Build history of the part. All positions in model axes, mm. Face numbers are marked on the shaded views. A direction names the side the tool comes from. Round coordinates to 2 decimals unless told otherwise and drop trailing zeros. Write each loop counter-clockwise with the first axis right and the second up, starting at its lowest first coordinate (ties: lowest second). Pieces come first, ordered by that corner, then holes. Notation, with made-up numbers: (14, 12) - (38, 12) arc R16 ccw to (38, 25) - close; hole circle Ø4 at (16.25, 69). An arc over 180 degrees is marked (long way). Write each question's results on one line, items separated by ' | '.
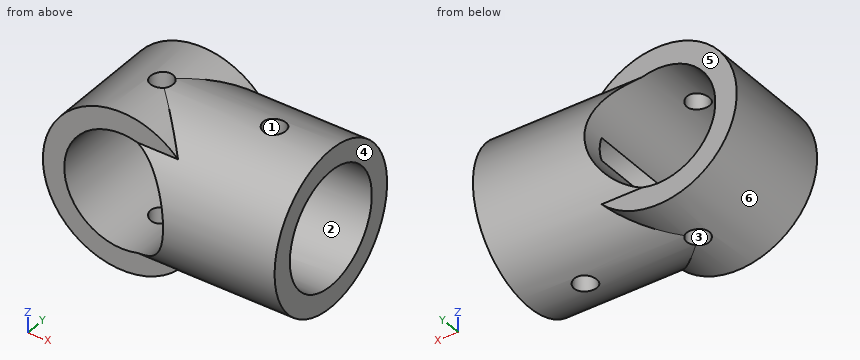
from build123d import *

# Parameters (mm, degrees)
CYLINDER001_R          = 10.2
CYLINDER001_DEPTH      = 20
CYLINDER002_R          = 2
CYLINDER002_DEPTH      = 30
CYLINDER003_R          = 2
CYLINDER003_DEPTH      = 30
CYLINDER_R             = 10.2
CYLINDER_DEPTH         = 30
CYLINDER_ROLL_ANGLE    = -90
CYLINDER004_R          = 14
CYLINDER004_DEPTH      = 30
CYLINDER005_R          = 14
CYLINDER005_DEPTH      = 20
CYLINDER005_ROLL_ANGLE = -90


with BuildPart() as cylinder001:
    # Cylinder001 → Cylinder001 (new body)
    with BuildSketch(Plane(origin=(10, 0, 0), x_dir=(0, -1, 0), z_dir=(1, 0, 0))):
        Circle(CYLINDER001_R)
    extrude(amount=CYLINDER001_DEPTH)


with BuildPart() as cylinder002:
    # Cylinder002 → Cylinder002 (new body)
    with BuildSketch(Plane.XY.offset(-15)):
        Circle(CYLINDER002_R)
    extrude(amount=CYLINDER002_DEPTH)


with BuildPart() as cylinder003:
    # Cylinder003 → Cylinder003 (new body)
    with BuildSketch(Plane(origin=(20, 0, -15), x_dir=(1, 0, 0), z_dir=(0, 0, 1))):
        Circle(CYLINDER003_R)
    extrude(amount=CYLINDER003_DEPTH)


with BuildPart() as negative_fusion:
    # Cylinder → Cylinder (new body)
    with BuildSketch(Plane.XY):
        Circle(CYLINDER_R)
    extrude(amount=CYLINDER_DEPTH)


with BuildPart() as negative_fusion_1:
    # Cylinder roll: moved
    add(negative_fusion.part.rotate(Axis((0, 0, 0), (1, 0, 0)), CYLINDER_ROLL_ANGLE))


with BuildPart() as negative_fusion_2:
    # Cylinder placement: moved
    add(negative_fusion_1.part.moved(Location((0, -15, 0))))

    # Fusion: union Cylinder001, Cylinder002, Cylinder003
    add(cylinder001.part)
    add(cylinder002.part)
    add(cylinder003.part)


with BuildPart() as cylinder004:
    # Cylinder004 → Cylinder004 (new body)
    with BuildSketch(Plane(origin=(0, 0, 0), x_dir=(0, -1, 0), z_dir=(1, 0, 0))):
        Circle(CYLINDER004_R)
    extrude(amount=CYLINDER004_DEPTH)


with BuildPart() as cut:
    # Cylinder005 → Cylinder005 (new body)
    with BuildSketch(Plane.XY):
        Circle(CYLINDER005_R)
    extrude(amount=CYLINDER005_DEPTH)


with BuildPart() as cut_1:
    # Cylinder005 roll: moved
    add(cut.part.rotate(Axis((0, 0, 0), (1, 0, 0)), CYLINDER005_ROLL_ANGLE))


with BuildPart() as cut_2:
    # Cylinder005 placement: moved
    add(cut_1.part.moved(Location((0, -10, 0))))

    # Fusion001: union Cylinder004
    add(cylinder004.part)

    # Cut: cut Negative Fusion
    add(negative_fusion_2.part, mode=Mode.SUBTRACT)


solid = cut_2.part
(1) Slice it at D-D, the plane z = -11. Write the cut outline in (x, y), and give its area (3 significant figures).
Worked answers:
outline: (-8.66, -10) - (8.66, -10) - (8.66, -8.66) - (30, -8.66) - (30, 8.66) - (8.66, 8.66) - (8.66, 10) - (-8.66, 10) - close; hole circle Ø4 at (0, 0); hole circle Ø4 at (20, 0) | area: 691 mm2
(2) Slice it at C-C, the plane y = 0. Write the cut outline in (x, z), and give its area (3 significant figures).
Worked answers:
outline: (-2, -13.86) - (-2, -10) arc R10.2 cw to (-2, 10) - (-2, 13.86) arc R14 ccw to start; (2, -14) - (18, -14) - (18, -10.2) - (10, -10.2) - (10, -2.01) arc R10.2 cw to (2, -10) - close; (2, 10) arc R10.2 cw to (10, 2.01) - (10, 10.2) - (18, 10.2) - (18, 14) - (2, 14) - close; (22, -14) - (30, -14) - (30, -10.2) - (22, -10.2) - close; (22, 10.2) - (30, 10.2) - (30, 14) - (22, 14) - close | area: 352 mm2
(3) Drill centre lines: probe 1 along Z at (x, y) = (15.5, 0); probe 2 along X at (y, z) = (0, -11.8); probe 3 along X at (y, z) = (0, -12). Where is each one in solid material? Low to high. Write a range as [from, to].
Worked answers:
probe 1: z = [-14, -10.2], [10.2, 14] | probe 2: x = [-7.53, -2], [2, 18], [22, 30] | probe 3: x = [-7.21, -2], [2, 18], [22, 30]
(4) Two-plate mould, pull along X, no slides. Class the marked faces 3, 4, 5 and 6: released by +X, released by -X, zero draft, split by the parting line, or undercut.
Worked answers:
face 3: undercut | face 4: released by +X | face 5: zero draft | face 6: split by the parting line
(5) Tool access for the marked faces 1 and 2: list every direction of +Z, -Z, +X, -X, +Y, -Y with a clear straight run to the whole face (end or side of a thin tool).
Worked answers:
face 1: +Z, -Z | face 2: +X
(6) Slice it at A-A, the plane z = 0. Write the cut outline in (x, y).
Worked answers:
outline: (-14, -10) - (-10.2, -10) - (-10.2, 10) - (-14, 10) - close; (10.2, -14) - (30, -14) - (30, -10.2) - (10.2, -10.2) - close; (10.2, 10.2) - (30, 10.2) - (30, 14) - (10.2, 14) - close
(7) Slice it at B-B, the plane x = 0. Write the cut outline in (y, z).
Worked answers:
outline: (-10, -14) - (-2, -14) - (-2, -10.2) - (-10, -10.2) - close; (-10, 10.2) - (-2, 10.2) - (-2, 14) - (-10, 14) - close; (2, -14) - (10, -14) - (10, -10.2) - (2, -10.2) - close; (2, 10.2) - (10, 10.2) - (10, 14) - (2, 14) - close
(8) Flat gauge pins, fed straight in: pin 1 Ø16.5 at (x, z) = (0, 0) entering from -Y; pin 2 Ø2 at (y, z) = (-4.5, -1.5) entering from -X; pin 3 Ø7 at (x, z) = (-6.5, -3) entering from -Y; pin 4 Ø5 at (x, z) = (-6.5, 7) entering from +Y. Where does each tip first touch, or does it go through?
Worked answers:
pin 1: passes through | pin 2: stops at x = -13.99 | pin 3: stops at y = -10 | pin 4: stops at y = 10
